Could you check a few things on this drawing? It's one solid part, dimensions in mm from its lowest x, y, z. A direction names the side the tool comes from. Round coordinates to 2 decimals unless told otherwise and drop trailing zeros. Order: outer loops, then holes, each group sorted by start corner. A loop starts at its lowest first (then second) coordinate and runs counter-clockwise, first axis right, second up.
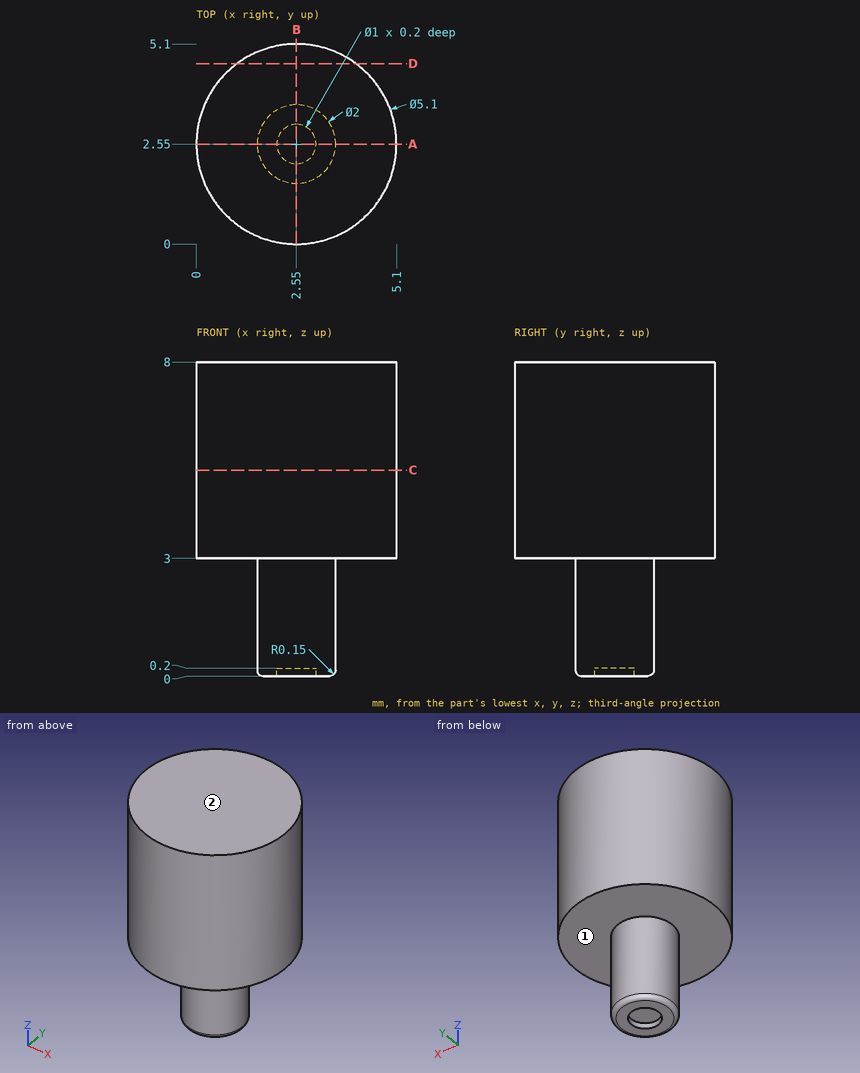
(1) Please list where these lines run through material, in increasing order: probe 1 along Y at (x, z) = (2.55, 0.15); probe 2 along Z at (x, y) = (0.9, 2); probe 3 along X at (y, z) = (1.1, 6.75).
(2) On a 3-axis mill with a long thin cutter (end or side, diameter ignored), from which of +Z, -Z, +X, -X, +Y, -Y can I reach the whole of each face in a straight line? I mean the marked faces 1 and 2. Say none if no direction works.
(3) I want a section at C-C, the plane z = 5.25. List the corners of the cut face in (x, y) for me.
(4) I want a section at D-D, the plane y = 4.6. List the corners of the cut face in (x, z) for me.
(5) I'm going to push a flat-ended pin straight in: pin 1 Ø1 at (x, z) = (0.5, 2) entering from +Y. Where does the tip first touch, or does it pass through?
(6) I want a section at A-A, the plane y = 2.55. List the corners of the cut face in (x, z) for me.
Ans:
1. probe 1: y = 1.55 to 2.05, 3.05 to 3.55
1. probe 2: z = 3 to 8
1. probe 3: x = 0.45 to 4.65
2. face 1: -Z
2. face 2: +Z, +X, -X, +Y, -Y
3. outline: circle Ø5.1 at (2.55, 2.55)
4. outline: (1.03, 3) - (4.07, 3) - (4.07, 8) - (1.03, 8) - close
5. pin 1: passes through
6. outline: (0, 3) - (1.55, 3) - (1.55, 0.15) arc R0.15 ccw to (1.7, 0) - (2.05, 0) - (2.05, 0.2) - (3.05, 0.2) - (3.05, 0) - (3.4, 0) arc R0.15 ccw to (3.55, 0.15) - (3.55, 3) - (5.1, 3) - (5.1, 8) - (0, 8) - close
